Part model, mm, in its own coordinate system. A direction names the side the tool comes from. Give positions to 0.01 mm unless a question says otherwise; leave off trailing zeros. Write each loop counter-clockwise with the first axis right and the second up, starting at its lowest first coordinate (ties: lowest second). Pieces come first, ordered by that corner, then holes.
Solid Edge part; units mm, degrees
sketch "Sketch1" plane through (0, 0, 8) normal (0, 0, 1) x (1, 0, 0)
  arc A0 (11.5046, 132.1857) -> (9.5064, 134.1) centre (9.5064, 132.1) ccw
  line L0 (9.5064, 134.1) -> (-18.7, 134.1)
  line L1 (-18.7, 134.1) -> (-18.7, 135.1)
  line L2 (9.4353, 135.1) -> (-18.7, 135.1)
  arc A1 (9.4353, 135.1) -> (13.5564, 136.4417) centre (9.4353, 142.1) ccw
  line L3 (13.5, 112.4) -> (21.002, 130.2247)
  line L4 (10.5, 112.4) -> (13.5, 112.4)
  line L5 (10.5, 122.9) -> (10.5, 112.4)
  arc A2 (7.5, 125.9) -> (10.5, 122.9) centre (7.5, 122.9) cw
  line L6 (-18.7, 125.9) -> (7.5, 125.9)
  line L7 (-18.7, 129.9) -> (-18.7, 125.9)
  line L8 (9.5179, 129.9) -> (-18.7, 129.9)
  arc A3 (9.5179, 129.9) -> (11.5128, 132.0429) centre (9.5179, 131.9) ccw
  arc A4 (11.5128, 132.0429) -> (11.5046, 132.1857) centre (16.5, 132.4) cw
  arc A5 (13.5564, 136.4417) -> (21.002, 130.2247) centre (16.5, 132.4) cw
  circle A6 centre (16.5, 132.4) radius 1.7
extrude "Protrusion1" add sketch "Sketch1" along normal up to vertex (3 mm away)
sketch "Sketch2" plane through (2.7972, 126.9, 11) normal (0, 0, 1) x (0, 1, 0)
  line L0 (-14.5, -10.7028) -> (-4.5, -10.7028)
  line L1 (-4.5, -10.7028) -> (-4.5, -7.7028)
  line L2 (-4.5, -7.7028) -> (-14.5, -7.7028)
  line L3 (-14.5, -7.7028) -> (-14.5, -10.7028)
  dimension "D1" = 4.5
  dimension "D2" = 14.5
extrude "Protrusion2" add sketch "Sketch2" along normal blind 7
sketch "Sketch3" plane through (12, 122.4, 14.5) normal (0, 1, 0) x (0, 0, -1)
  line L0 (3.5, -4.4705) -> (3.5, -1.5)
  line L1 (3.5, -1.5) -> (-3.5, -1.5)
  line L2 (-3.5, -1.5) -> (3.5, -4.4705)
extrude "ExtrudedProtrusion_3" add sketch "Sketch3" against normal blind 2
sketch "Sketch4" plane through (1.4, 124.9, 11) normal (0, 0, 1) x (1, 0, 0)
  line L0 (-10.1, 1) -> (-10.1, 5)
  line L1 (-10.1, 5) -> (-20.1, 5)
  line L2 (-20.1, 5) -> (-20.1, 1)
  line L3 (-20.1, 1) -> (-10.1, 1)
extrude "ExtrudedProtrusion_4" add sketch "Sketch4" along normal blind 3
fillet "Round_1" radius 3 1 edges at (-8.7, 127.9, 11)
sketch "Sketch5" plane through (-13.7, 127.9, 14) normal (0, 0, 1) x (1, 0, 0)
  line L0 (24.2, -7.0304) -> (24.2, -5)
  arc A0 (24.2, -5) -> (19.2, 0) centre (19.2, -5) ccw
  line L1 (19.2, 0) -> (-6.0361, 0)
extrude "Cutout1" cut sketch "Sketch5" against normal through all material side at (10.45, 121.8848, 14)
1) Flat gauge pins, fed straight in: P1, Ø3, axis at x = -2, z = 10, coming from the +Y side; P2, Ø7.5, axis at x = 1, y = 127.5, coming from the +Z side; P3, Ø1.6, axis at x = -12.5, y = 128.5, coming from the +Z side. Where does each tip first touch, or does it go through?
Check result:
P1: stops at y = 135.1
P2: stops at z = 11
P3: stops at z = 14
2) 3-axis set-ups, long thin cutter, end or side, ignore diameter. For faces 1 (the flat face through (-9, 127.9, 10)), 2 (the flat face through (-4, 134.1, 9)), 3 (the flat face through (14, 120.4, 13)): which of +Z, -Z, +X, -X, +Y, -Y reach the whole face in a straight line?
Check result:
face 1: +Z, -Z, -X, -Y
face 2: +Z, -Z, -X
face 3: +Z, +X, -Y
3) Saw through at A-A (x = -15.5). Write the cut outline in (y, z), and give its area (3 significant figures).
Check result:
outline: (127.9, 8) - (129.9, 8) - (129.9, 14) - (127.9, 14) - close; (134.1, 8) - (135.1, 8) - (135.1, 11) - (134.1, 11) - close
area: 15.0 mm2
4) Saw through at C-C (x = -2.5). Write the cut outline in (y, z).
Check result:
outline: (127.9, 8) - (129.9, 8) - (129.9, 11) - (127.9, 11) - close; (134.1, 8) - (135.1, 8) - (135.1, 11) - (134.1, 11) - close
5) Saw through at D-D (z = 9.75). Write the cut outline in (x, y).
Check result:
outline: (-18.7, 127.9) - (5.5, 127.9) arc R5 cw to (10.5, 122.9) - (10.5, 112.4) - (13.5, 112.4) - (21, 130.22) arc R5 ccw to (13.56, 136.44) arc R7 cw to (9.44, 135.1) - (-18.7, 135.1) - (-18.7, 134.1) - (9.51, 134.1) arc R2 cw to (11.5, 132.19) arc R5 ccw to (11.51, 132.04) arc R2 cw to (9.52, 129.9) - (-18.7, 129.9) - close; hole circle Ø3.4 at (16.5, 132.4)
6) Drill centre lines: L1, parallel to X at y = 132.4, z = 9.9; L2, parallel to Z at x = -10, y = 128.75; L3, parallel to Z at x = 12, y = 132.5. Where is each one in solid material? Low to high.
Check result:
L1: x = 11.48 to 14.8, 18.2 to 21.5
L2: z = 8 to 14
L3: z = 8 to 11
7) Mould opens along Y. For faces 4 (the flat face through (-8, 129.9, 10)), 5 (the flat face through (12, 112.4, 13)), 6 (the cylindrical face through (16.13, 134.06, 9.48)), 7 (the flat face through (-4, 135.1, 9)) say: +Y half, -Y half, draft (parallel to the pull), parting line (faces both ways), or undercut.
Check result:
face 4: undercut
face 5: -Y half
face 6: undercut
face 7: +Y half
8) Saw through at B-B (z = 11.75). Write the cut outline in (x, y).
Check result:
outline: (-18.7, 127.9) - (-7.68, 127.9) - (-7.68, 129.9) - (-18.7, 129.9) - close; (10.5, 112.4) - (13.5, 112.4) - (13.5, 120.4) - (16.15, 120.4) - (16.15, 122.4) - (10.5, 122.4) - close
